Work out the finished part from the listing and answer in its coordinate system (mm). A direction names the side the tool comes from. Round coordinates to 2 decimals unless told otherwise and drop trailing zeros. Order: outer loops, then holes, each group sorted by start corner. A loop starts at its lowest first (then second) coordinate and runs counter-clockwise, first axis right, second up. Notation, with made-up numbers: M -24,13 L -5,13 A30 ccw -5,48 Z; hole C 16.5,-19.75 d8. An arc over 180 degrees is marked long. Return JSON: item names as keys, results as strings.
from build123d import *

# Parameters (mm, degrees)
CUT_EXTRUDE1_DEPTH = 17
SKETCH3_W          = 12
SKETCH3_H          = 16
CHAMFER1_SIZE2     = 1.000000021
CHAMFER1_SIZE      = 1.000000018
CHAMFER2_SIZE      = 0.5
SCALE1_SCALE       = 0.3


with BuildPart() as part:
    # Sketch1 → Revolve1 (revolve)
    with BuildSketch(Plane(origin=(0, 0, 0), x_dir=(1, 0, 0), z_dir=(0, 1, 0))):
        Polygon((43, 8), (0, 8), (0, -8), (43, -8), (43, -6.003672577), (32, -2), (32, 2), (43, 6.003672577), align=None)
    revolve(axis=Axis((0, 0, -8), (0, 0, 1)))

    # Sketch2 → Cut-Extrude1 (cut, through all)
    with BuildSketch(Plane.XY.offset(8)):
        with BuildLine():
            Line((-15, -4), (-11.313708499, -4))
            ThreePointArc((-11.313708499, -4), (-12, -1e-09), (-11.313708499, 3.999999999))
            Line((-11.313708499, 3.999999999), (-15, 3.999999999))
            Line((-15, 3.999999999), (-15, -4))
        make_face()
    extrude(amount=-CUT_EXTRUDE1_DEPTH, mode=Mode.SUBTRACT)

    # Sketch3 → Cut-Revolve1 (revolve, cut)
    with BuildSketch(Plane(origin=(0, 0, 0), x_dir=(1, 0, 0), z_dir=(0, 1, 0))):
        with Locations((6, 0)):
            Rectangle(SKETCH3_W, SKETCH3_H)
    revolve(axis=Axis((0, 0, -8), (0, 0, 1)), mode=Mode.SUBTRACT)

    # Chamfer1
    chamfer1_edges = [part.edges().sort_by_distance(p)[0] for p in [
        (12, 1e-09, -8),
        (12, 1e-09, 8),
    ]]
    chamfer(chamfer1_edges, length=CHAMFER1_SIZE, length2=CHAMFER1_SIZE2)

    # Chamfer2
    chamfer2_edges = [part.edges().sort_by_distance(p)[0] for p in [
        (-43, 0, 8),
        (-43, 0, -8),
    ]]
    chamfer(chamfer2_edges, length=CHAMFER2_SIZE)


with BuildPart() as part_1:
    # Scale1: scaled about (0.084922045, 0, 0)
    add(part.part.scale(SCALE1_SCALE).moved(Location((0.059445431, 0, 0))))


solid = part_1.part
Item 1: Consider line 1 along Z through (x, y) = (-7.5, -6.5); line 2 along Y through (x, z) = (2.25, 0.4); line 3 along Z through (x, y) = (-8.5, 6.25). Determine where each line is inside the solid, lowest interval first. Write a range as [from, to].
Output:
{"line 1": "z = [-2.4, -0.73], [0.73, 2.4]", "line 2": "y = [-9.35, -2.86], [2.86, 9.35]", "line 3": "z = [-2.4, -0.96], [0.96, 2.4]"}
Item 2: Which of the six approach directions +Z, -Z, +X, -X, +Y, -Y give full straight-line access (tool end or side, diameter ignored) to faces 4 (the conical face through (3.771, -0.147, -2.215)), 5 (the flat face through (-4, 1.2, 0)), 6 (the conical face through (9.413, 2.946, -0.675))?
Output:
{"face 4": "-Z", "face 5": "+Z, -Z", "face 6": "none"}
Item 3: Find section A-A (y = 0). Determine the outline of the cut face in (x, z).
Output:
{"outline": "M -12.84,-2.25 L -12.69,-2.4 L -4.44,-2.4 L -4.44,2.4 L -12.69,2.4 L -12.84,2.25 L -12.84,1.8 L -9.54,0.6 L -9.54,-0.6 L -12.84,-1.8 Z; M 3.66,-2.1 L 3.96,-2.4 L 12.81,-2.4 L 12.96,-2.25 L 12.96,-1.8 L 9.66,-0.6 L 9.66,0.6 L 12.96,1.8 L 12.96,2.25 L 12.81,2.4 L 3.96,2.4 L 3.66,2.1 Z"}
Item 4: The mould has two halves that part along Y. Classify faces 1 (the flat face through (-3, 3, 2.4)), 2 (the flat face through (-4.441, 0, 0)), 3 (the conical face through (-2.06, -9.53, 0.66)): pulls with the +Y half, pulls with the -Y half, needs draft (parallel to the pull), parting line crosses it, or undercut.
Output:
{"face 1": "needs draft", "face 2": "undercut", "face 3": "parting line crosses it"}
